Source: CAD feature listing. Evaluate the final solid. Frame: model axes, mm. Coordinates: 2 decimals unless noted, no trailing zeros. Write each loop counter-clockwise with the first axis right and the second up, starting at its lowest first coordinate (ties: lowest second). Pieces come first, ordered by that corner, then holes. Notation, with made-up numbers: M -11.75,68 L 28.25,68 A21 cw 28.25,100 Z; hole C 24,9 d9. An arc over 180 degrees is marked long. Write item = value, one per line. Start each with the question number.
1. Section query C-C (z = 93.6). Output: boundary loops of the cut face in (x, y), then the cut area to 3 significant figures.
2. Section query A-A (x = 0). Output: boundary loops of the cut face in (y, z), then the cut area to 3 significant figures.
3. Line query: line 1 along X through (y, z) = (2.5, 49.85); line 2 along X through (y, z) = (3.5, -6.15); line 3 along Z through (x, y) = (15, 2.5). Output: solid intervals per line, ascending.
4. Section query B-B (z = -93.6). Output: boundary loops of the cut face in (x, y), then the cut area to 3 significant figures.
5. Section query D-D (y = 3.75). Give the number of separate pieces and of enclosed holes in the cut face, then the cut area to 3 significant figures.
```python
from build123d import *
from OCP.BRepFilletAPI import BRepFilletAPI_MakeChamfer

# Parameters (mm, degrees)
ESQUISSE1_W              = 203.2
ESQUISSE1_H              = 203.2
BOSS_EXTRU_1_DEPTH       = 6.35
ESQUISSE2_R              = 2.5
ENL_V_MAT_EXTRU_1_DEPTH  = 144.824345992
ESQUISSE3_R              = 2.5
ENL_V_MAT_EXTRU_2_DEPTH  = 144.824345992
ESQUISSE4_R              = 2.5
ENL_V_MAT_EXTRU_3_DEPTH  = 144.824345992
ESQUISSE6_R              = 2.5
ENL_V_MAT_EXTRU_5_DEPTH  = 144.824345992
ENL_V_MAT_EXTRU_9_DEPTH  = 144.824345992
ENL_V_MAT_EXTRU_4_DEPTH  = 144.824345992
ENL_V_MAT_EXTRU_7_DEPTH  = 144.824345992
ENL_V_MAT_EXTRU_8_DEPTH  = 144.824345992
CONG_2_R                 = 4
ESQUISSE12_R             = 2.6
ENL_V_MAT_EXTRU_10_DEPTH = 144.824345992
CHANFREIN2_SIZE          = 7
CHANFREIN2_SIZE2         = 12.124355653
CHANFREIN3_SIZE          = 7
CHANFREIN3_SIZE2         = 12.124355653


with BuildPart() as part:
    # Esquisse1 → Boss.-Extru.1 (new body)
    with BuildSketch(Plane(origin=(0, 0, 0), x_dir=(1, 0, 0), z_dir=(0, 1, 0))):
        Rectangle(ESQUISSE1_W, ESQUISSE1_H)
    extrude(amount=BOSS_EXTRU_1_DEPTH)

    # Esquisse2 → Enlèv. mat.-Extru.1 (cut, through all)
    with BuildSketch(Plane(origin=(0, 6.35, 0), x_dir=(1, 0, 0), z_dir=(0, 1, 0))):
        with Locations(Location((-35.6, -49.85, 0), (0, 0, 270))):
            Circle(ESQUISSE2_R)
        with Locations(Location((-35.6, -79.85, 0), (0, 0, 270))):
            Circle(ESQUISSE2_R)
        with Locations(Location((35.9, -79.85, 0), (0, 0, 270))):
            Circle(ESQUISSE2_R)
        with Locations(Location((35.9, -49.85, 0), (0, 0, 270))):
            Circle(ESQUISSE2_R)
    extrude(amount=-ENL_V_MAT_EXTRU_1_DEPTH, mode=Mode.SUBTRACT)

    # Esquisse3 → Enlèv. mat.-Extru.2 (cut, through all)
    with BuildSketch(Plane(origin=(0, 6.35, 0), x_dir=(1, 0, 0), z_dir=(0, 1, 0))):
        with Locations(Location((-93.6, 93.6, 0), (0, 0, 270))):
            Circle(ESQUISSE3_R)
        with Locations(Location((93.6, 93.6, 0), (0, 0, 270))):
            Circle(ESQUISSE3_R)
        with Locations(Location((93.6, -93.6, 0), (0, 0, 270))):
            Circle(ESQUISSE3_R)
        with Locations(Location((-93.6, -93.6, 0), (0, 0, 270))):
            Circle(ESQUISSE3_R)
    extrude(amount=-ENL_V_MAT_EXTRU_2_DEPTH, mode=Mode.SUBTRACT)

    # Esquisse4 → Enlèv. mat.-Extru.3 (cut, through all)
    with BuildSketch(Plane(origin=(0, 6.35, 0), x_dir=(1, 0, 0), z_dir=(0, 1, 0))):
        with Locations(Location((15.588457268, 56, 0), (0, 0, 270))):
            Circle(ESQUISSE4_R)
        with Locations(Location((-15.588457268, 56, 0), (0, 0, 270))):
            Circle(ESQUISSE4_R)
        with Locations(Location((0, 83, 0), (0, 0, 270))):
            Circle(ESQUISSE4_R)
        with Locations(Location((-75, -83, 0), (0, 0, 270))):
            Circle(ESQUISSE4_R)
        with Locations(Location((-90.588457268, -56, 0), (0, 0, 270))):
            Circle(ESQUISSE4_R)
        with Locations(Location((-59.411542732, -56, 0), (0, 0, 270))):
            Circle(ESQUISSE4_R)
        with Locations(Location((59.413008586, -55.999154304, 0), (0, 0, 270))):
            Circle(ESQUISSE4_R)
        with Locations(Location((90.589923123, -55.999154304, 0), (0, 0, 270))):
            Circle(ESQUISSE4_R)
        with Locations(Location((75.001465855, -82.999154304, 0), (0, 0, 270))):
            Circle(ESQUISSE4_R)
    extrude(amount=-ENL_V_MAT_EXTRU_3_DEPTH, mode=Mode.SUBTRACT)

    # Esquisse6 → Enlèv. mat.-Extru.5 (cut, through all)
    with BuildSketch(Plane.XZ):
        with Locations(Location((-56, 85, 0), (0, 0, 270))):
            Circle(ESQUISSE6_R)
        with Locations(Location((-56, -85, 0), (0, 0, 270))):
            Circle(ESQUISSE6_R)
        with Locations(Location((-82, 0, 0), (0, 0, 270))):
            Circle(ESQUISSE6_R)
    enl_v_mat_extru_5 = extrude(amount=-ENL_V_MAT_EXTRU_5_DEPTH, mode=Mode.SUBTRACT)

    # Symétrie1: Enlèv. mat.-Extru.5 across plane
    add(enl_v_mat_extru_5.mirror(Plane(origin=(0, 0, 0), x_dir=(0, 0, 1), z_dir=(1, 0, 0))), mode=Mode.SUBTRACT)

    # Esquisse11 → Enlèv. mat.-Extru.9 (cut, through all)
    with BuildSketch(Plane(origin=(0, 6.35, 0), x_dir=(1, 0, 0), z_dir=(0, 1, 0))):
        Polygon((-16.978069991, 42.150000003), (16.978069991, 42.150000003), (21.15, 37.978069994), (21.15, 4.021930012), (16.978069991, -0.149999997), (-16.978069991, -0.149999997), (-21.15, 4.021930012), (-21.15, 37.978069994), align=None)
    extrude(amount=-ENL_V_MAT_EXTRU_9_DEPTH, mode=Mode.SUBTRACT)

    # Esquisse5 → Enlèv. mat.-Extru.4 (cut, through all)
    with BuildSketch(Plane(origin=(0, 6.35, 0), x_dir=(1, 0, 0), z_dir=(0, 1, 0))):
        Polygon((3.651740453, -4), (-3.651740453, -4), (-7.303480905, -10.325), (-3.651740453, -16.65), (3.651740453, -16.65), (7.303480905, -10.325), align=None)
    extrude(amount=-ENL_V_MAT_EXTRU_4_DEPTH, mode=Mode.SUBTRACT)

    # Esquisse9 → Enlèv. mat.-Extru.7 (cut, through all)
    with BuildSketch(Plane(origin=(0, 6.35, 0), x_dir=(1, 0, 0), z_dir=(0, 1, 0))):
        Polygon((-16.978069991, -43.85), (16.978069991, -43.85), (21.15, -48.021930009), (21.15, -81.978069991), (16.978069991, -86.15), (-16.978069991, -86.15), (-21.15, -81.978069991), (-21.15, -48.021930009), align=None)
    extrude(amount=-ENL_V_MAT_EXTRU_7_DEPTH, mode=Mode.SUBTRACT)

    # Esquisse10 → Enlèv. mat.-Extru.8 (cut, through all)
    with BuildSketch(Plane(origin=(0, 6.35, 0), x_dir=(1, 0, 0), z_dir=(0, 1, 0))):
        Polygon((21.15, -58.928069991), (42.1, -58.928069991), (42.1, 15.071930012), (21.15, 15.071930012), (21.15, 27.071930012), (49.6, 27.071930012), (49.6, 15.071930012), (49.6, -58.928069991), (49.6, -70.928069991), (49.6, -101.6), (42.1, -101.6), (42.1, -70.928069991), (21.15, -70.928069991), align=None)
    extrude(amount=-ENL_V_MAT_EXTRU_8_DEPTH, mode=Mode.SUBTRACT)

    # Congé2
    cong_2_edges = [part.edges().sort_by_distance(p)[0] for p in [
        (42.1, 3.175, 58.928069991),
        (42.1, 3.175, -15.071930012),
        (49.6, 3.175, -27.071930012),
        (49.6, 3.175, 101.6),
        (42.1, 3.175, 101.6),
        (42.1, 3.175, 70.928069991),
        (101.6, 3.175, 101.6),
        (-101.6, 3.175, 101.6),
        (-101.6, 3.175, -101.6),
        (101.6, 3.175, -101.6),
    ]]
    fillet(cong_2_edges, radius=CONG_2_R)

    # Esquisse12 → Enlèv. mat.-Extru.10 (cut, through all)
    with BuildSketch(Plane(origin=(0, 6.35, 0), x_dir=(1, 0, 0), z_dir=(0, 1, 0))):
        with Locations(Location((-35.6, 36.15, 0), (0, 0, 270))):
            Circle(ESQUISSE12_R)
        with Locations(Location((-35.6, 6.15, 0), (0, 0, 270))):
            Circle(ESQUISSE12_R)
        with Locations(Location((35.9, 6.15, 0), (0, 0, 270))):
            Circle(ESQUISSE12_R)
        with Locations(Location((35.9, 36.15, 0), (0, 0, 270))):
            Circle(ESQUISSE12_R)
    extrude(amount=-ENL_V_MAT_EXTRU_10_DEPTH, mode=Mode.SUBTRACT)

    # Chanfrein2: one chamfer whose edges measure the first distance from different faces: ONE call of the kernel's chamfer builder (chamfer() names one face for all edges)
    chanfrein2_edges_1 = [part.edges().sort_by_distance(p)[0] for p in [
        (21.15, 3.175, 70.928069991),
    ]]
    chanfrein2_side_1 = [part.faces().sort_by_distance(p)[0] for p in [
        (21.15, 3.175, 76.453069991),
    ]]
    chanfrein2_edges_2 = [part.edges().sort_by_distance(p)[0] for p in [
        (21.15, 3.175, 58.928069991),
    ]]
    chanfrein2_side_2 = [part.faces().sort_by_distance(p)[0] for p in [
        (21.15, 3.175, 53.475),
    ]]
    chanfrein2 = BRepFilletAPI_MakeChamfer(part.part.solid().wrapped)
    for e in chanfrein2_edges_1:
        chanfrein2.Add(CHANFREIN2_SIZE, CHANFREIN2_SIZE2, e.wrapped, chanfrein2_side_1[0].wrapped)  # the first distance lies on this face
    for e in chanfrein2_edges_2:
        chanfrein2.Add(CHANFREIN2_SIZE, CHANFREIN2_SIZE2, e.wrapped, chanfrein2_side_2[0].wrapped)  # the first distance lies on this face
    add(Compound.cast(chanfrein2.Shape()), mode=Mode.REPLACE)

    # Chanfrein3: one chamfer whose edges measure the first distance from different faces: ONE call of the kernel's chamfer builder (chamfer() names one face for all edges)
    chanfrein3_edges_1 = [part.edges().sort_by_distance(p)[0] for p in [
        (21.15, 3.175, -15.071930012),
    ]]
    chanfrein3_side_1 = [part.faces().sort_by_distance(p)[0] for p in [
        (21.15, 3.175, -9.546930012),
    ]]
    chanfrein3_edges_2 = [part.edges().sort_by_distance(p)[0] for p in [
        (21.15, 3.175, -27.071930012),
    ]]
    chanfrein3_side_2 = [part.faces().sort_by_distance(p)[0] for p in [
        (21.15, 3.175, -32.525000003),
    ]]
    chanfrein3 = BRepFilletAPI_MakeChamfer(part.part.solid().wrapped)
    for e in chanfrein3_edges_1:
        chanfrein3.Add(CHANFREIN3_SIZE, CHANFREIN3_SIZE2, e.wrapped, chanfrein3_side_1[0].wrapped)  # the first distance lies on this face
    for e in chanfrein3_edges_2:
        chanfrein3.Add(CHANFREIN3_SIZE, CHANFREIN3_SIZE2, e.wrapped, chanfrein3_side_2[0].wrapped)  # the first distance lies on this face
    add(Compound.cast(chanfrein3.Shape()), mode=Mode.REPLACE)


solid = part.part
```
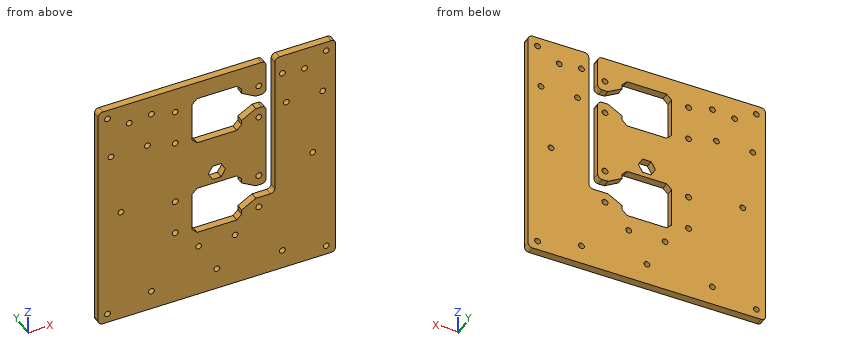
Results are:
q1.outline = M -101.6,0 L -96.1,0 L -96.1,6.35 L -101.6,6.35 Z; M -91.1,0 L 42.1,0 L 42.1,6.35 L -91.1,6.35 Z; M 49.6,0 L 91.1,0 L 91.1,6.35 L 49.6,6.35 Z; M 96.1,0 L 101.6,0 L 101.6,6.35 L 96.1,6.35 Z
q1.area = 1,180 mm^2
q2.outline = M 0,-101.6 L 6.35,-101.6 L 6.35,-85.5 L 0,-85.5 Z; M 0,-80.5 L 6.35,-80.5 L 6.35,-42.15 L 0,-42.15 Z; M 0,0.15 L 6.35,0.15 L 6.35,4 L 0,4 Z; M 0,16.65 L 6.35,16.65 L 6.35,43.85 L 0,43.85 Z; M 0,86.15 L 6.35,86.15 L 6.35,101.6 L 0,101.6 Z
q2.area = 641 mm^2
q3.line_1 = -101.6 to -38.1, -33.1 to -21.15, 21.15 to 33.4, 38.4 to 42.1, 49.6 to 101.6
q3.line_2 = -101.6 to -38.2, -33 to -21.15, 21.15 to 33.3, 38.5 to 42.1, 49.6 to 101.6
q3.line_3 = -101.6 to -58.43, -53.57 to -42.15, 0.15 to 43.85, 86.15 to 101.6
q4.outline = M -101.6,0 L -96.1,0 L -96.1,6.35 L -101.6,6.35 Z; M -91.1,0 L 91.1,0 L 91.1,6.35 L -91.1,6.35 Z; M 96.1,0 L 101.6,0 L 101.6,6.35 L 96.1,6.35 Z
q4.area = 1,230 mm^2
q5.separate_pieces = 1
q5.enclosed_holes = 28
q5.area = 35,400 mm^2
